Verification items for the finished model (mm, model axes). A direction names the side the tool comes from. Coordinates: 2 decimals unless noted, no trailing zeros. Order: outer loops, then holes, each group sorted by start corner. A loop starts at its lowest first (then second) coordinate and runs counter-clockwise, first axis right, second up. Notation, with made-up numbers: (25.5, 50.25) -> (40.5, 50.25) arc R32 cw to (40.5, 81.25) -> close; hole circle Ø4 at (-10.5, 10). An arc over 180 degrees is marked (long way). Use CSV: the item, a comma, the result in double quotes. Start each with the question number.
1) Go/stop test with flat-tipped pins: pin 1 (1.4 mm diameter, centred on x = 32, z = 80, fed in from -Y); pin 2 (2 mm diameter, centred on x = -32, z = 0, fed in from +Y); pin 3 (6.5 mm diameter, centred on x = 8, z = -6, fed in from +Y). Record where each tip stops, or that it passes through.
2) Release check for a two-part mould opening along X. For faces 5 (the cylindrical face through (-45.1, 9.8, 26.2)), 6 (the flat face through (0, 9, 85)) record: released by +X, released by -X, zero draft, split by the parting line, or undercut.
3) Sectioned sample at A-A on y = 5.75. Record the boundary of the cut face in (x, z).
4) Sectioned sample at B-B on z = 2.5. Record the boundary of the cut face in (x, y).
5) Sectioned sample at C-C on x = 15. Record the boundary of the cut face in (y, z).
6) Scan lines: line 1 along X through (y, z) = (0.7, 48); line 2 along Z through (x, y) = (-34, 9.75); line 3 along Y through (x, z) = (-35.5, 68.5). Record each from-to range of solid material in increasing order.
7) Tool access check on faces 1 (the flat face through (39.2, 7.4, 79.2)), 2 (the cylindrical face through (45.1, 9.8, 53.8)), 3 (the cylindrical face through (-24, 9.8, -5.1)), 4 (the flat face through (42, 12, 1)). Record the directions out of +Z, -Z, +X, -X, +Y, -Y that give a thin tool (end or side, any length) a straight path to the whole face; none if there is none.
from build123d import *

# Parameters (mm, degrees)
SKETCH1_W           = 96
SKETCH1_H           = 96
SKETCH1_R           = 0.75
BOSS_EXTRUDE1_DEPTH = 3
SKETCH2_W           = 96
SKETCH2_H           = 96
BOSS_EXTRUDE2_DEPTH = 9
SKETCH3_R           = 1.5
CUT_EXTRUDE1_DEPTH  = 9
CUT_EXTRUDE2_DEPTH  = 109
CUT_EXTRUDE3_DEPTH  = 131.782261794
SKETCH6_R           = 0.75
CUT_EXTRUDE4_DEPTH  = 101.642933185
LPATTERN4_COUNT     = 3
LPATTERN4_PITCH     = 32


with BuildPart() as part:
    # Sketch1 → Boss-Extrude1 (new body)
    with BuildSketch(Plane(origin=(0, 0, 0), x_dir=(1, 0, 0), z_dir=(0, 1, 0))):
        with Locations((0, -40)):
            Rectangle(SKETCH1_W, SKETCH1_H)
        with Locations(Location((0, 0, 0), (0, 0, 270))):
            Circle(SKETCH1_R, mode=Mode.SUBTRACT)
        with Locations(Location((32, 0, 0), (0, 0, 270))):
            Circle(SKETCH1_R, mode=Mode.SUBTRACT)
        with Locations(Location((-32, 0, 0), (0, 0, 270))):
            Circle(SKETCH1_R, mode=Mode.SUBTRACT)
        with Locations(Location((0, -16, 0), (0, 0, 270))):
            Circle(SKETCH1_R, mode=Mode.SUBTRACT)
        with Locations(Location((-32, -16, 0), (0, 0, 270))):
            Circle(SKETCH1_R, mode=Mode.SUBTRACT)
        with Locations(Location((32, -16, 0), (0, 0, 270))):
            Circle(SKETCH1_R, mode=Mode.SUBTRACT)
        with Locations(Location((0, -32, 0), (0, 0, 270))):
            Circle(SKETCH1_R, mode=Mode.SUBTRACT)
        with Locations(Location((-32, -32, 0), (0, 0, 270))):
            Circle(SKETCH1_R, mode=Mode.SUBTRACT)
        with Locations(Location((32, -32, 0), (0, 0, 270))):
            Circle(SKETCH1_R, mode=Mode.SUBTRACT)
        with Locations(Location((0, -48, 0), (0, 0, 270))):
            Circle(SKETCH1_R, mode=Mode.SUBTRACT)
        with Locations(Location((-32, -48, 0), (0, 0, 270))):
            Circle(SKETCH1_R, mode=Mode.SUBTRACT)
        with Locations(Location((32, -48, 0), (0, 0, 270))):
            Circle(SKETCH1_R, mode=Mode.SUBTRACT)
        with Locations(Location((0, -64, 0), (0, 0, 270))):
            Circle(SKETCH1_R, mode=Mode.SUBTRACT)
        with Locations(Location((-32, -64, 0), (0, 0, 270))):
            Circle(SKETCH1_R, mode=Mode.SUBTRACT)
        with Locations(Location((32, -64, 0), (0, 0, 270))):
            Circle(SKETCH1_R, mode=Mode.SUBTRACT)
        with Locations(Location((0, -80, 0), (0, 0, 270))):
            Circle(SKETCH1_R, mode=Mode.SUBTRACT)
        with Locations(Location((-32, -80, 0), (0, 0, 270))):
            Circle(SKETCH1_R, mode=Mode.SUBTRACT)
        with Locations(Location((32, -80, 0), (0, 0, 270))):
            Circle(SKETCH1_R, mode=Mode.SUBTRACT)
    extrude(amount=BOSS_EXTRUDE1_DEPTH)

    # Sketch2 → Boss-Extrude2 (add)
    with BuildSketch(Plane(origin=(0, 3, 0), x_dir=(1, 0, 0), z_dir=(0, 1, 0))):
        with Locations((0, -40)):
            Rectangle(SKETCH2_W, SKETCH2_H)
        Polygon((-36.2, 2.2), (36.2, 2.2), (42.2, -3.8), (42.2, -76.2), (36.2, -82.2), (-36.2, -82.2), (-42.2, -76.2), (-42.2, -3.8), align=None, mode=Mode.SUBTRACT)
    extrude(amount=BOSS_EXTRUDE2_DEPTH)

    # Sketch3 → Cut-Extrude1 (cut)
    with BuildSketch(Plane(origin=(0, 12, 0), x_dir=(1, 0, 0), z_dir=(0, 1, 0))):
        with Locations(Location((-42.2, 2.2, 0), (0, 0, 270))):
            Circle(SKETCH3_R)
        with Locations(Location((42.2, 2.2, 0), (0, 0, 270))):
            Circle(SKETCH3_R)
        with Locations(Location((42.2, -82.2, 0), (0, 0, 270))):
            Circle(SKETCH3_R)
        with Locations(Location((-42.2, -82.2, 0), (0, 0, 270))):
            Circle(SKETCH3_R)
    extrude(amount=-CUT_EXTRUDE1_DEPTH, mode=Mode.SUBTRACT)

    # Sketch4 → Cut-Extrude2 (cut, through all)
    with BuildSketch(Plane.XY.offset(88)):
        with BuildLine():
            Line((-26.2, 12), (26.2, 12))
            ThreePointArc((26.2, 12), (24.003847577, 9.803847577), (21.003847577, 9))
            Line((21.003847577, 9), (-21.003847577, 9))
            ThreePointArc((-21.003847577, 9), (-24.003847577, 9.803847577), (-26.2, 12))
        make_face()
    extrude(amount=-CUT_EXTRUDE2_DEPTH, mode=Mode.SUBTRACT)

    # Sketch5 → Cut-Extrude3 (cut, through all)
    with BuildSketch(Plane.ZY.offset(48)):
        with BuildLine():
            Line((29.196152423, 9), (50.803847577, 9))
            ThreePointArc((50.803847577, 9), (53.803847577, 9.803847577), (56, 12))
            Line((56, 12), (24, 12))
            ThreePointArc((24, 12), (26.196152423, 9.803847577), (29.196152423, 9))
        make_face()
    extrude(amount=-CUT_EXTRUDE3_DEPTH, mode=Mode.SUBTRACT)

    # Sketch6 → Cut-Extrude4 (cut, through all)
    with BuildSketch(Plane(origin=(0, 3, 0), x_dir=(1, 0, 0), z_dir=(0, 1, 0))):
        with Locations(Location((-30, -72, 0), (0, 0, 270))):
            Circle(SKETCH6_R)
    cut_extrude4 = extrude(amount=-CUT_EXTRUDE4_DEPTH, mode=Mode.SUBTRACT)

    # LPattern4: Cut-Extrude4 ×3
    with Locations(*[(0, 0, -i * LPATTERN4_PITCH) for i in range(1, LPATTERN4_COUNT)]):
        add(cut_extrude4, mode=Mode.SUBTRACT)


solid = part.part
Answers follow:
1,pin 1,"passes through"
1,pin 2,"stops at y = 3"
1,pin 3,"stops at y = 9"
2,face 5,"zero draft"
2,face 6,"undercut"
3,outline,"(-48, -8) -> (48, -8) -> (48, 88) -> (-48, 88) -> close; hole circle Ø3 at (-42.2, -2.2); hole circle Ø3 at (-42.2, 82.2); hole (-42.2, 3.8) -> (-36.2, -2.2) -> (36.2, -2.2) -> (42.2, 3.8) -> (42.2, 76.2) -> (36.2, 82.2) -> (-36.2, 82.2) -> (-42.2, 76.2) -> close; hole circle Ø3 at (42.2, -2.2); hole circle Ø3 at (42.2, 82.2)"
4,outline,"(-48, 0) -> (48, 0) -> (48, 12) -> (40.9, 12) -> (40.9, 3) -> (-40.9, 3) -> (-40.9, 12) -> (-48, 12) -> close"
5,outline,"(0, -8) -> (9, -8) -> (9, -2.2) -> (3, -2.2) -> (3, 82.2) -> (9, 82.2) -> (9, 88) -> (0, 88) -> close"
6,line 1,"x = -48 to -32.75, -31.25 to -0.75, 0.75 to 31.25, 32.75 to 48"
6,line 2,"z = -8 to -2.2, 82.2 to 88"
6,line 3,"y = 0 to 3"
7,face 1,"+Y"
7,face 2,"+X, -X, +Y"
7,face 3,"+Z, -Z, +Y"
7,face 4,"+Z, -Z, +X, -X, +Y"
